```python
from build123d import *

# Parameters (mm, degrees)
F0_W      = 59.2034347355
F0_H      = 39.4279696047
F1_DEPTH  = 50.8
F2_T      = -2.54
F3_W      = 12.1403969824
F3_H      = 8.035345003
F3_W_2    = 12.169610709
F3_H_2    = 8.255334571
F3_W_3    = 12.2919734567
F3_H_3    = 8.0133527517
F3_W_4    = 11.809963733
F3_H_4    = 6.7030247301
F4_DEPTH  = 304.8
F5_W      = 25.1509935988
F5_H      = 33.6675519442
F5_W_2    = 35.1178152452
F5_H_2    = 32.8409761062
F6_DEPTH  = 25.4
F7_W      = 19.4892128929
F7_H      = 32.6723456383
F8_DEPTH  = 25.4
F10_DEPTH = 44.958
F12_DEPTH = 45.974
F14_DEPTH = 38.1
F16_W     = 22.1592243761
F16_H     = 29.5382153708
F17_DEPTH = 5.08
F18_W     = 2.54
F18_H     = 51.3208392394
F19_DEPTH = 48.768
F20_W     = 54.1234347355
F20_H     = 2.6716254652
F21_DEPTH = 48.514


with BuildPart() as f1:
    # F0 (on Top) → F1 (new body)
    with BuildSketch(Plane.XY):
        Polygon((59.2034347355, 56.4008392394), (-55.2182495594, 56.4008392394), (-55.2182495594, 0), (0, 0), (59.2034347355, 0), align=None)
        with Locations((29.6017173678, -19.7139848024)):
            Rectangle(F0_W, F0_H)
    extrude(amount=F1_DEPTH)

    # F2
    f2_openings = [f1.faces().sort_by_distance(p)[0] for p in [
        (9.326345, 15.473019, 50.8),
    ]]
    offset(amount=F2_T, openings=f2_openings, kind=Kind.INTERSECTION)

    # F3 (on Front) → F4 (cut)
    with BuildSketch(Plane.XZ):
        with Locations((-37.3727958649, 33.3452494815)):
            Rectangle(F3_W, F3_H)
        with Locations((-21.8836758286, 33.4552442655)):
            Rectangle(F3_W_2, F3_H_2)
        with Locations((-21.9448572025, 22.8410381824)):
            Rectangle(F3_W_3, F3_H_3)
        with Locations((-37.2075792402, 22.1858741716)):
            Rectangle(F3_W_4, F3_H_4)
    extrude(amount=-F4_DEPTH, mode=Mode.SUBTRACT)

    # F5 (on face) → F6 (cut)
    with BuildSketch(Plane.YZ.offset(59.2034347355)):
        with Locations((-11.6124728053, 24.9852682464)):
            Rectangle(F5_W, F5_H)
        with Locations((23.6019316167, 24.5719803274)):
            Rectangle(F5_W_2, F5_H_2)
    extrude(amount=-F6_DEPTH, mode=Mode.SUBTRACT)

    # F7 (on face) → F8 (join)
    with BuildSketch(Plane.XZ.offset(39.4279696047)):
        with Locations((23.9334818907, 16.3361728191)):
            Rectangle(F7_W, F7_H)
    extrude(amount=F8_DEPTH)

    # F9 (on face) → F10 (cut)
    with BuildSketch(Plane.XY.offset(32.6723456383)):
        Polygon((14.1888754442, -42.09953174), (14.1888754442, -64.8279696047), (31.4645133913, -64.8279696047), align=None)
    extrude(amount=-F10_DEPTH, mode=Mode.SUBTRACT)

    # F11 (on face) → F12 (cut)
    with BuildSketch(Plane.XY.offset(32.6723456383)):
        Polygon((15.7361254096, -39.4279696047), (33.6780883372, -63.2997527719), (33.6780883372, -39.4279696047), align=None)
    extrude(amount=-F12_DEPTH, mode=Mode.SUBTRACT)

    # F13 (on face) → F14 (cut)
    with BuildSketch(Plane.XY.offset(32.6723456383)):
        Polygon((33.6780883372, -63.2997527719), (31.4645133913, -64.8279696047), (33.6780883372, -64.8279696047), align=None)
    extrude(amount=-F14_DEPTH, mode=Mode.SUBTRACT)

    # F16 (on face) → F17 (cut)
    with BuildSketch(Plane.XZ.offset(39.4279696047)):
        with Locations((27.4216728285, 17.1910146018)):
            Rectangle(F16_W, F16_H)
    extrude(amount=-F17_DEPTH, mode=Mode.SUBTRACT)

    # F18 (on face) → F19 (join)
    with BuildSketch(Plane.XY.offset(2.54)):
        with Locations((1.27, 28.2004196197)):
            Rectangle(F18_W, F18_H)
    extrude(amount=F19_DEPTH)

    # F20 (on face) → F21 (join)
    with BuildSketch(Plane.XY.offset(2.54)):
        with Locations((29.6017173678, 1.3358127326)):
            Rectangle(F20_W, F20_H)
    extrude(amount=F21_DEPTH)


solid = f1.part
```
Here's how the part is built. I have some questions about the finished solid (model axes, mm). A direction names the side the tool comes from. Give positions to 0.01 mm unless a question says otherwise; leave off trailing zeros. Order: outer loops, then holes, each group sorted by start corner. A loop starts at its lowest first (then second) coordinate and runs counter-clockwise, first axis right, second up. Notation, with made-up numbers: (73.25, 30.5) - (123.25, 30.5) arc R8 ccw to (123.25, 43.5) - close; hole circle Ø2 at (37.25, 70.5). An arc over 180 degrees is marked (long way). Answer as a JSON object with one key per item and string values. Group by question number.
Item 1: If we section it at D-D on x = 11: Please give me the cut outline in (y, z), and give its area (3 significant figures).
Item 2: If we section it at A-A on x = -18: Please give me the cut outline in (y, z), and give its area (3 significant figures).
Item 3: If we section it at B-B on z = 6: Please give me the cut outline in (x, y).
Item 4: If we mould it in two halves opening along Y, with no side actions, what happens to faces 1 (the flat face through (22.948, -53.623, 16.565)), 2 (the flat face through (-3, 2, 50.8)), 3 (the flat face through (56.663, -27, 26))? For each: pulls with the +Y half, pulls with the -Y half, needs draft (parallel to the pull), parting line crosses it, or undercut.
Item 5: Which directions (+Z, -Z, +X, -X, +Y, -Y) give clear straight access to the entire face, cutting with the end or side of a thin tool? Please do faces 4 (the flat face through (38.501, -38, 17)), 5 (the flat face through (24.582, -51.197, 16.565)), 6 (the flat face through (30, 53.861, 26)), 7 (the flat face through (23, -52, 32.672)).
Item 6: For P1, Ø1, axis at y = -33, z = 29, coming from the -X side; P2, Ø2, axis at y = -52.5, z = 13.5, coming from the +X side; P3, Ø6, axis at y = -16, z = 19, coming from the +X side, each with a flat end and sliding along its axis, tell me the tip position at first contact or that it passes through.
Item 7: Please list where these lines run through material, in increasing order: probe 1 along Y at (x, z) = (39, 23); probe 2 along X at (y, z) = (51, 37); probe 3 along X at (y, z) = (-33, 28).
Item 8: If we section it at C-C on y = -14: Please give me the cut outline in (x, z).
Result set:
{
 "1": {"outline": "(-39.43, 0) - (56.4, 0) - (56.4, 50.8) - (53.86, 50.8) - (53.86, 2.54) - (2.67, 2.54) - (2.67, 51.05) - (0, 51.05) - (0, 2.54) - (-36.89, 2.54) - (-36.89, 50.8) - (-39.43, 50.8) - close", "area": "618 mm²"},
 "2": {"outline": "(0, 0) - (56.4, 0) - (56.4, 18.83) - (53.86, 18.83) - (53.86, 2.54) - (2.54, 2.54) - (2.54, 18.83) - (0, 18.83) - close; (0, 26.85) - (2.54, 26.85) - (2.54, 29.33) - (0, 29.33) - close; (0, 37.58) - (2.54, 37.58) - (2.54, 50.8) - (0, 50.8) - close; (53.86, 26.85) - (56.4, 26.85) - (56.4, 29.33) - (53.86, 29.33) - close; (53.86, 37.58) - (56.4, 37.58) - (56.4, 50.8) - (53.86, 50.8) - close", "area": "306 mm²"},
 "3": {"outline": "(-55.22, 0) - (0, 0) - (0, -39.43) - (14.19, -39.43) - (14.19, -42.1) - (31.46, -64.83) - (33.68, -63.3) - (15.74, -39.43) - (16.34, -39.43) - (16.34, -36.89) - (2.54, -36.89) - (2.54, 0) - (56.66, 0) - (56.66, -36.89) - (38.5, -36.89) - (38.5, -39.43) - (59.2, -39.43) - (59.2, 56.4) - (-55.22, 56.4) - close; hole (-52.68, 2.54) - (0, 2.54) - (0, 53.86) - (-52.68, 53.86) - close; hole (2.54, 2.67) - (56.66, 2.67) - (56.66, 53.86) - (2.54, 53.86) - close"},
 "4": {"face 1": "pulls with the -Y half", "face 2": "needs draft", "face 3": "undercut"},
 "5": {"face 4": "-Y", "face 5": "+Z, -Z, +X", "face 6": "+Z", "face 7": "+Z, +X, -X, -Y"},
 "6": {"P1": "x = 0", "P2": "x = 26.31", "P3": "x = 2.54"},
 "7": {"probe 1": "-39.43 to -36.89, 0 to 2.67, 53.86 to 56.4", "probe 2": "-55.22 to -52.68, 0 to 2.54, 56.66 to 59.2", "probe 3": "0 to 2.54, 56.66 to 59.2"},
 "8": {"outline": "(0, 0) - (59.2, 0) - (59.2, 8.15) - (56.66, 8.15) - (56.66, 2.54) - (2.54, 2.54) - (2.54, 50.8) - (0, 50.8) - close; (56.66, 41.82) - (59.2, 41.82) - (59.2, 50.8) - (56.66, 50.8) - close"}
}
